For this review, take the finished solid that the model builds, in its own axes (mm). Coordinates: 2 decimals unless noted, no trailing zeros. Order: outer loops, then holes, each group sorted by start corner. A loop starts at its lowest first (then second) coordinate and runs counter-clockwise, first axis right, second up. Notation, with made-up numbers: (45.25, -6) -> (101.25, -6) arc R29 ccw to (101.25, 17) -> close; hole circle Ø4 at (-8, -26.75). An arc over 180 degrees is marked (long way). Return JSON: item names as keys, results as strings. Group by question number.
Item 1: For line 1 along Z through (x, y) = (-0.5, -9); line 2 along Y through (x, z) = (18.5, -12); line 3 along Z through (x, y) = (-7.5, -19.5), list the stretches that pass through material, from the lowest coordinate up.
Item 2: Take a section at A-A (z = 0). Write out the cut boundary in (x, y) (3 decimals).
Item 3: Insertion check: pin 1 (3 mm diameter, centred on y = -16.5, z = 25, fed in from -X); pin 2 (10 mm diameter, centred on x = 25.5, y = -13.5, fed in from +Z); pin 3 (12 mm diameter, centred on x = -4, y = -17.5, fed in from +Z). Each pin has a flat end and moves straight along its axis. Give the tip position at first contact, or say it passes through.
Item 4: Draft analysis for pull direction X (two halves, no side actions). For faces 1 (the flat face through (0, -25.4, 0)), 2 (the cylindrical face through (31.5, -13.5, 9.9)), 3 (the flat face through (0, 0, 0)), state which applies: +X half, -X half, draft (parallel to the pull), parting line (faces both ways), or undercut.
```python
from build123d import *

# Parameters (mm, degrees)
F0_R     = 33.02
F0_R_2   = 28.575
F1_DEPTH = 27.94
F2_DEPTH = 25.4


# Not quite as in the source:
# - a fillet or chamfer that OpenCascade refuses, or shapes differently, is made with other operations: its cross-section is extruded or revolved along the edge and cut away or added


with BuildPart() as f1:
    # F0 (on Front) → F1 (new body)
    with BuildSketch(Plane.XZ):
        Circle(F0_R)
        Circle(F0_R_2, mode=Mode.SUBTRACT)
    extrude(amount=F1_DEPTH)

    # F0 (on Front) → F2 (join)
    with BuildSketch(Plane.XZ):
        Circle(F0_R_2)
        with BuildLine():
            add(Edge.make_bspline(
                [(-8.89, -23.495), (-8.89, -31.1939658396), (4.445, -27.3444829198), (17.78, -23.495), (4.445, -19.6455170802), (-8.89, -15.7960341604), (-8.89, -23.495)],
                knots=[0, 0, 0, 2.0943951024, 2.0943951024, 4.1887902048, 4.1887902048, 6.2831853072, 6.2831853072, 6.2831853072], degree=2, weights=[1, 0.5, 1, 0.5, 1, 0.5, 1]))
        make_face(mode=Mode.SUBTRACT)
    extrude(amount=F2_DEPTH)

    # F3: chamfer of 5.08 on 1 edges, made by hand


with BuildPart() as f3_tool2:
    # F3_s3 → F3_t4 (revolve)
    with BuildSketch(Plane.XY):
        Polygon((33.655, -27.94), (28.575, -22.86), (28.575, -27.94), align=None)
    revolve(axis=Axis((0, -27.94, 0), (0, -1, 0)))

    split(bisect_by=Plane.XZ.offset(25.4), keep=Keep.TOP)


with BuildPart() as f1_1:
    add(f1.part)

    # F3_t1: cut F3_tool2
    add(f3_tool2.part, mode=Mode.SUBTRACT)


solid = f1_1.part
```
Findings below:
{
 "1": {"line 1": "z = -33.02 to -27.93, -19.06 to 33.02", "line 2": "y = -25.4 to 0", "line 3": "z = -32.16 to -25.88, -21.11 to 32.16"},
 "2": {"outline": "(-33.02, -27.305) -> (-31.115, -25.4) -> (31.115, -25.4) -> (33.02, -27.305) -> (33.02, 0) -> (-33.02, 0) -> close"},
 "3": {"pin 1": "stops at x = -23.2", "pin 2": "stops at z = 25.89", "pin 3": "stops at z = 33.02"},
 "4": {"face 1": "undercut", "face 2": "parting line", "face 3": "draft"}
}
